from build123d import *

# Parameters (mm, degrees)
SKETCH1_W           = 33.02
SKETCH1_H           = 29.21
BOSS_EXTRUDE1_DEPTH = 6.35
CUT_EXTRUDE1_REACH  = 24.939
SKETCH3_R           = 3.175
SKETCH3_W           = 6.35
SKETCH3_H           = 19.05
SKETCH3_W_2         = 20.8534
SKETCH3_H_2         = 5.08
FILLET1_R           = 10.16
FILLET2_R           = 2.54


with BuildPart() as part:
    # Sketch1 → Boss-Extrude1 (new body)
    with BuildSketch(Plane.XY):
        Rectangle(SKETCH1_W, SKETCH1_H)
    extrude(amount=BOSS_EXTRUDE1_DEPTH)

    # Sketch3 → Cut-Extrude1 (cut, up to next)
    with BuildSketch(Plane.XY.offset(6.35), mode=Mode.PRIVATE) as cut_extrude1_sk1:
        with Locations((0, 4.445)):
            Circle(SKETCH3_R)
    cut_extrude1_tool1 = extrude(cut_extrude1_sk1.sketch, amount=-CUT_EXTRUDE1_REACH, mode=Mode.PRIVATE) & part.part
    # Sketch3 → Cut-Extrude1 (cut, up to next)
    with BuildSketch(Plane.XY.offset(6.35), mode=Mode.PRIVATE) as cut_extrude1_sk2:
        with Locations((-13.335, 5.08)):
            Rectangle(SKETCH3_W, SKETCH3_H)
    cut_extrude1_tool2 = extrude(cut_extrude1_sk2.sketch, amount=-CUT_EXTRUDE1_REACH, mode=Mode.PRIVATE) & part.part
    # Sketch3 → Cut-Extrude1 (cut, up to next)
    with BuildSketch(Plane.XY.offset(6.35), mode=Mode.PRIVATE) as cut_extrude1_sk3:
        with Locations((13.335, 5.08)):
            Rectangle(SKETCH3_W, SKETCH3_H)
    cut_extrude1_tool3 = extrude(cut_extrude1_sk3.sketch, amount=-CUT_EXTRUDE1_REACH, mode=Mode.PRIVATE) & part.part
    # Sketch3 → Cut-Extrude1 (cut, up to next)
    with BuildSketch(Plane.XY.offset(6.35), mode=Mode.PRIVATE) as cut_extrude1_sk4:
        with Locations((0, -12.065)):
            Rectangle(SKETCH3_W_2, SKETCH3_H_2)
    cut_extrude1_tool4 = extrude(cut_extrude1_sk4.sketch, amount=-CUT_EXTRUDE1_REACH, mode=Mode.PRIVATE) & part.part
    add(cut_extrude1_tool1.solids().sort_by_distance((0, 4.445, 6.35))[0], mode=Mode.SUBTRACT)
    add(cut_extrude1_tool2.solids().sort_by_distance((-13.335, 5.08, 6.35))[0], mode=Mode.SUBTRACT)
    add(cut_extrude1_tool3.solids().sort_by_distance((13.335, 5.08, 6.35))[0], mode=Mode.SUBTRACT)
    add(cut_extrude1_tool4.solids().sort_by_distance((0, -12.065, 6.35))[0], mode=Mode.SUBTRACT)

    # Fillet1
    fillet1_edges = [part.edges().sort_by_distance(p)[0] for p in [
        (10.16, 14.605, 3.175),
        (-10.16, 14.605, 3.175),
    ]]
    fillet(fillet1_edges, radius=FILLET1_R - 0.0001)  # a hair under: the kernel refuses the full size

    # Fillet2
    fillet2_edges = [part.edges().sort_by_distance(p)[0] for p in [
        (10.16, -4.445, 3.175),
        (-10.4267, -9.525, 3.175),
        (10.4267, -9.525, 3.175),
        (-10.16, -4.445, 3.175),
    ]]
    fillet(fillet2_edges, radius=FILLET2_R)


solid = part.part
Check sheet for the modelled part. Datum: model origin and axes. Units: mm. A direction names the side the tool comes from. Coordinates: 2 decimals unless noted, no trailing zeros. Loops run counter-clockwise (first coordinate to the right, second up) from the corner with the lowest first, then second, coordinate; pieces in that order, holes last. Notation, with made-up numbers: (26.5, 82) -> (67.5, 82) arc R14 cw to (67.5, 95) -> close; hole circle Ø7 at (-39.75, 87.25). An arc over 180 degrees is marked (long way). Answer in a Markdown table with one row per item.
1. Sectioned sample at D-D, the plane x = -11. Record the boundary of the cut face in (y, z) (3 decimals).
Check values:
| item | result |
|---|---|
| outline | (-14.605, 0) -> (-3.792, 0) -> (-3.792, 6.35) -> (-14.605, 6.35) -> close |
2. Material ranges on line 1 along Y through (x, z) = (0, 4.5) (3 decimals); line 2 along X through (y, z) = (-0.75, 5.5); line 3 along X through (y, z) = (5.5, 2.5), recorded low to high. Write a range as [from, to].
Check values:
| item | result |
|---|---|
| line 1 | y = [-9.525, 1.27], [7.62, 14.605] |
| line 2 | x = [-10.16, 10.16] |
| line 3 | x = [-10.11, -2.99], [2.99, 10.11] |
3. Sectioned sample at A-A, the plane x = -1. Record the boundary of the cut face in (y, z) (3 decimals).
Check values:
| item | result |
|---|---|
| outline | (-9.525, 0) -> (1.432, 0) -> (1.432, 6.35) -> (-9.525, 6.35) -> close; (7.458, 0) -> (14.556, 0) -> (14.556, 6.35) -> (7.458, 6.35) -> close |
4. Sectioned sample at B-B, the plane y = -11.25. Record the boundary of the cut face in (x, z).
Check values:
| item | result |
|---|---|
| outline | (-16.51, 0) -> (-10.29, 0) -> (-10.29, 6.35) -> (-16.51, 6.35) -> close; (10.29, 0) -> (16.51, 0) -> (16.51, 6.35) -> (10.29, 6.35) -> close |
5. Release check for a two-part mould opening along X. For faces 4 (the face through (-16.51, -10, 3)), 5 (the face through (0, -9.525, 3)), 6 (the face through (10.884, -3.681, 3.131)) record: released by +X, released by -X, zero draft, split by the parting line, or undercut.
Check values:
| item | result |
|---|---|
| face 4 | released by -X |
| face 5 | undercut |
| face 6 | released by +X |
6. Access from +Z, -Z, +X, -X, +Y, -Y to the whole of each face (thin tool, end or side, straight path). Record for faces 1 (the face through (-15, -4.445, 3)), 2 (the face through (15, -4.445, 3)), 3 (the face through (-10.427, -13, 3)).
Check values:
| item | result |
|---|---|
| face 1 | +Z, -Z, -X, +Y |
| face 2 | +Z, -Z, +X, +Y |
| face 3 | +Z, -Z, -Y |
7. Go/stop test with flat-tipped pins: pin 1 (3 mm diameter, centred on x = 4.5, z = 3.5, fed in from -Y) (3 decimals); pin 2 (3 mm diameter, centred on y = 1, z = 2, fed in from +X); pin 3 (2 mm diameter, centred on y = 2.5, z = 5.5, fed in from -X). Record where each tip stops, or that it passes through.
Check values:
| item | result |
|---|---|
| pin 1 | stops at y = -9.525 |
| pin 2 | stops at x = 10.16 |
| pin 3 | stops at x = -10.16 |
